For this review, use the dimensioned drawing (mm, ordinates from the lowest corner) and the shaded views. A direction names the side the tool comes from. Give positions to 0.01 mm unless a question says otherwise; leave off trailing zeros. Write each loop counter-clockwise with the first axis right and the second up, starting at its lowest first coordinate (ties: lowest second). Pieces come first, ordered by that corner, then holes. Notation, with made-up numbers: M 33.25,82.5 L 85.25,82.5 A6 cw 85.25,88.5 Z; hole C 36,-7.5 d1. An arc over 180 degrees is marked long. One line per item, written item: value. Start each with the question number.
Item 1: Consider section C-C, the plane y = 35. Write out the cut boundary in (x, z), and give its area (3 significant figures).
Item 2: Consider section B-B, the plane x = 44.45. Write out the cut boundary in (y, z).
Item 3: To check wall thickness, follow probe 1 along X at (y, z) = (6, 114); probe 2 along Z at (x, y) = (12.7, 7); probe 3 along Z at (x, y) = (14.5, 6). State the ranges of each line that lie inside material, in increasing order.
Item 4: Consider section D-D, the plane x = 58.5. Write out the cut boundary in (y, z), and give its area (3 significant figures).
Item 5: Tool access review of the marked faces 4, 5 and 6: name each direction out of +Z, -Z, +X, -X, +Y, -Y from which nothing blocks a thin tool from reaching the whole face with its end or side.
Item 6: Mouldability with a two-part tool opening along Z and no side actions: class the marked faces 1, 2 and 3 as released by +Z, released by -Z, zero draft, split by the parting line, or undercut.
Item 7: Clearance check with flat-ended pins moving along their axes: pin 1 Ø5 at (y, z) = (54, 63) entering from +X; pin 2 Ø19 at (x, y) = (27.5, 31.5) entering from +Z; pin 3 Ø2 at (x, z) = (27, 37.5) entering from +Y. State where each tip first meets the part, or that it passes through.
Item 8: Consider section A-A, the plane z = 114.3. Write out the cut boundary in (x, y), and give its area (3 significant figures).
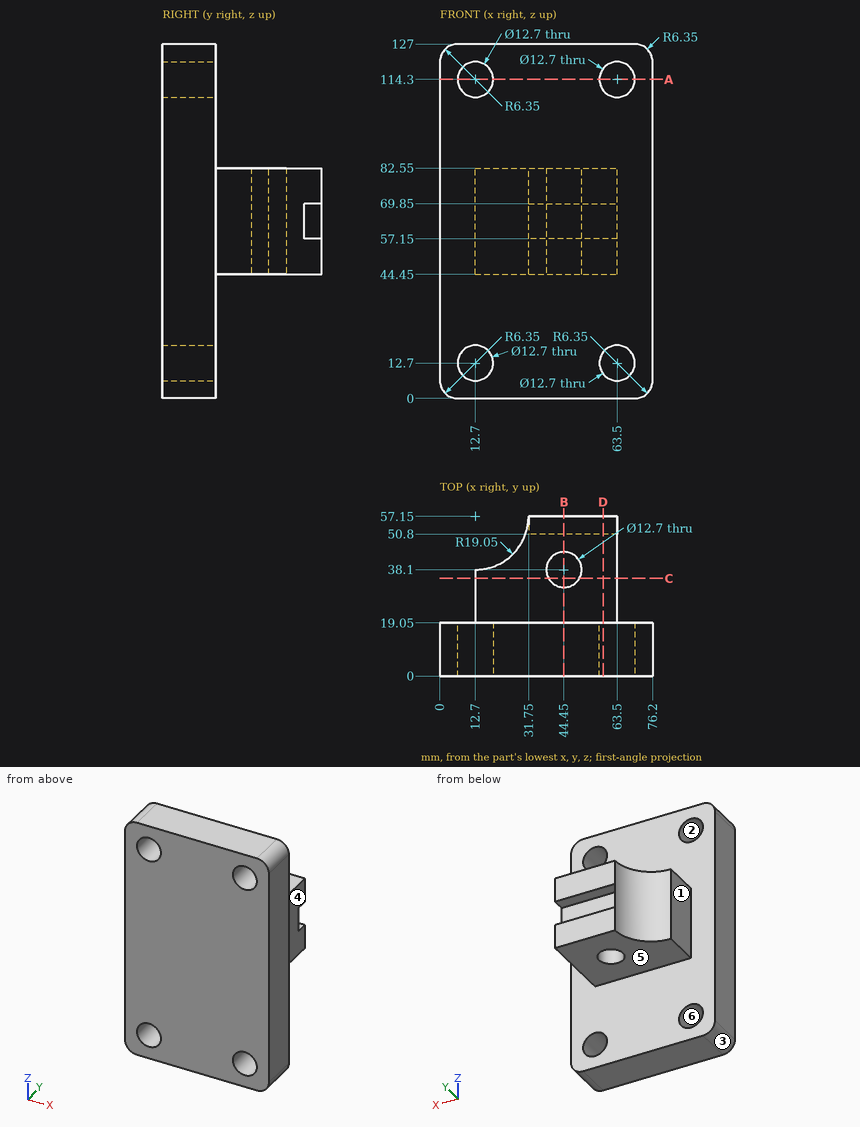
Model answer:
1. outline: M 12.7,44.45 L 38.91,44.45 L 38.91,82.55 L 12.7,82.55 Z; M 49.99,44.45 L 63.5,44.45 L 63.5,82.55 L 49.99,82.55 Z
1. area: 1,510 mm2
2. outline: M 0,0 L 19.05,0 L 19.05,44.45 L 31.75,44.45 L 31.75,82.55 L 19.05,82.55 L 19.05,127 L 0,127 Z; M 44.45,44.45 L 57.15,44.45 L 57.15,57.15 L 50.8,57.15 L 50.8,69.85 L 57.15,69.85 L 57.15,82.55 L 44.45,82.55 Z
3. probe 1: x = 0 to 6.36, 19.04 to 57.16, 69.84 to 76.2
3. probe 2: z = 0 to 6.35, 19.05 to 107.95, 120.65 to 127
3. probe 3: z = 0 to 6.61, 18.79 to 108.21, 120.39 to 127
4. outline: M 0,0 L 19.05,0 L 19.05,8.79 L 0,8.79 Z; M 0,16.61 L 19.05,16.61 L 19.05,44.45 L 57.15,44.45 L 57.15,57.15 L 50.8,57.15 L 50.8,69.85 L 57.15,69.85 L 57.15,82.55 L 19.05,82.55 L 19.05,110.39 L 0,110.39 Z; M 0,118.21 L 19.05,118.21 L 19.05,127 L 0,127 Z
4. area: 3,490 mm2
5. face 4: +Z, -Z, +X, +Y
5. face 5: -Z, +X, -X, +Y
5. face 6: +Y, -Y
6. face 1: zero draft
6. face 2: undercut
6. face 3: released by -Z
7. pin 1: stops at x = 31.75
7. pin 2: stops at z = 82.55
7. pin 3: stops at y = 19.05
8. outline: M 0,0 L 6.35,0 L 6.35,19.05 L 0,19.05 Z; M 19.05,0 L 57.15,0 L 57.15,19.05 L 19.05,19.05 Z; M 69.85,0 L 76.2,0 L 76.2,19.05 L 69.85,19.05 Z
8. area: 968 mm2
